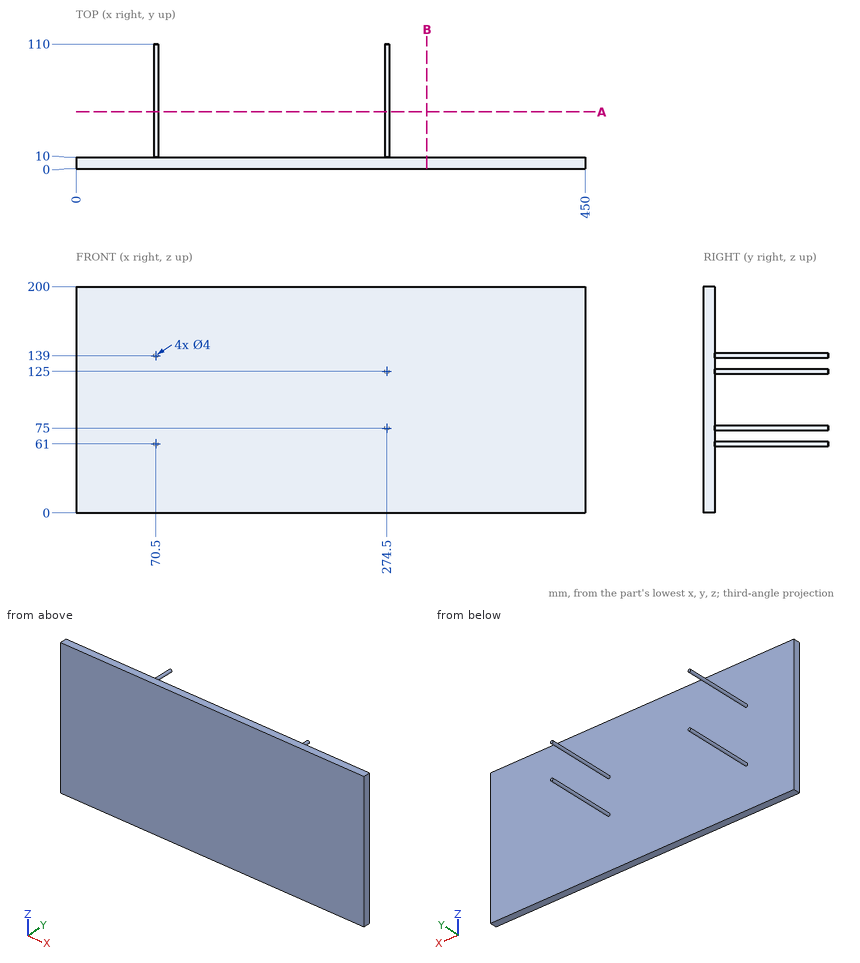
Here's the drawing with two shaded views (mm, measured from the low corner). I have some questions. Round coordinates to 2 decimals unless told otherwise and drop trailing zeros. Write each loop counter-clockwise with the first axis right and the second up, starting at its lowest first coordinate (ties: lowest second). Pieces come first, ordered by that corner, then holes. Notation, with made-up numbers: M 18.5,22.25 L 69.5,22.25 A15 ccw 69.5,35.25 Z; hole C 66.5,26.5 d7. An arc over 180 degrees is marked long. Write each question's results on one line, items separated by ' | '. Start each with the question number.
1. Imagine slicing it at B-B on x = 310. List the corners of the cut face in (y, z) for me, and give its area (3 significant figures).
2. Imagine slicing it at A-A on y = 50. List the corners of the cut face in (x, z) for me, and give its area (3 significant figures).
3. I'm going to push flat-ended pins straight in: pin 1 Ø8 at (x, z) = (102.5, 179.5) entering from +Y; pin 2 Ø12 at (x, z) = (209, 114) entering from -Y; pin 3 Ø10 at (y, z) = (17.5, 66) entering from +X. Where does each tip first touch, or does it pass through?
4. I need wall thicknesses on L1, parallel to Z at x = 71, y = 97; L2, parallel to Y at x = 76, z = 34.5. Which ranges of each line are inside material? Lowest first, please. Write a range as from..to.
Result sheet:
1) outline: M 0,0 L 10,0 L 10,200 L 0,200 Z | area: 2,000 mm^2
2) outline: C 70.5,61 d4; C 70.5,139 d4; C 274.5,75 d4; C 274.5,125 d4 | area: 50.3 mm^2
3) pin 1: stops at y = 10 | pin 2: stops at y = 0 | pin 3: stops at x = 72.5
4) L1: z = 59.06..62.94, 137.06..140.94 | L2: y = 0..10
